```python
from build123d import *

# Parameters (mm, degrees)
SKETCH1_R           = 1.25
SKETCH1_R_2         = 1.75
BOSS_EXTRUDE2_DEPTH = 5


with BuildPart() as part:
    # Sketch1 → Boss-Extrude2 (new body)
    with BuildSketch(Plane.XY):
        with BuildLine():
            Line((386.419721239, 336.571497364), (385.293365012, 338.860526411))
            Line((385.293365012, 338.860526411), (383.908113185, 336.571143013))
            Line((383.908113185, 336.571143013), (382.503747201, 338.700952515))
            Line((382.503747201, 338.700952515), (381.416354322, 336.256003497))
            Line((381.416354322, 336.256003497), (379.756126272, 338.193005085))
            Line((379.756126272, 338.193005085), (378.983741177, 335.631048754))
            Line((378.983741177, 335.631048754), (377.093833849, 337.344694757))
            Line((377.093833849, 337.344694757), (376.648637512, 334.706134696))
            Line((376.648637512, 334.706134696), (374.558855873, 336.169399891))
            Line((374.558855873, 336.169399891), (374.447869306, 333.495847767))
            Line((374.447869306, 333.495847767), (372.191170461, 334.685655589))
            Line((372.191170461, 334.685655589), (372.41614399, 332.019274917))
            Line((372.41614399, 332.019274917), (370.028117427, 332.916861386))
            Line((370.028117427, 332.916861386), (370.585503084, 330.299702582))
            Line((370.585503084, 330.299702582), (368.10380941, 330.890912222))
            Line((368.10380941, 330.890912222), (368.98481689, 328.364249444))
            Line((368.98481689, 328.364249444), (366.448593896, 328.639758526))
            Line((366.448593896, 328.639758526), (367.639329184, 326.243438755))
            Line((367.639329184, 326.243438755), (365.088574622, 326.198902337))
            Line((365.088574622, 326.198902337), (366.570259113, 323.970716967))
            Line((366.570259113, 323.970716967), (364.045199905, 323.606837414))
            Line((364.045199905, 323.606837414), (365.794466549, 321.58192626))
            Line((365.794466549, 321.58192626), (363.334924388, 320.904442171))
            Line((363.334924388, 320.904442171), (365.324186205, 319.114739291))
            Line((365.324186205, 319.114739291), (362.96894954, 318.134334994))
            Line((362.96894954, 318.134334994), (365.166834682, 316.608065071))
            Line((365.166834682, 316.608065071), (362.953047003, 315.340202129))
            Line((362.953047003, 315.340202129), (365.324893508, 314.101435352))
            Line((365.324893508, 314.101435352), (363.287467569, 312.566108719))
            Line((363.287467569, 312.566108719), (365.795870002, 311.63438118))
            Line((365.795870002, 311.63438118), (363.966937226, 309.855803875))
            Line((363.966937226, 309.855803875), (366.572336582, 309.245809474))
            Line((366.572336582, 309.245809474), (364.980740332, 307.252030724))
            Line((364.980740332, 307.252030724), (367.642047906, 306.973389437))
            Line((367.642047906, 306.973389437), (366.312888606, 304.795852323))
            Line((366.312888606, 304.795852323), (368.988133989, 304.85295849))
            Line((368.988133989, 304.85295849), (367.942373274, 302.526004073))
            Line((367.942373274, 302.526004073), (370.589366248, 302.917957095))
            Line((370.589366248, 302.917957095), (369.84349639, 300.478282837))
            Line((369.84349639, 300.478282837), (372.420492294, 301.198901382))
            Line((372.420492294, 301.198901382), (371.986276106, 298.684982403))
            Line((371.986276106, 298.684982403), (374.452634175, 299.722901884))
            Line((374.452634175, 299.722901884), (374.336919507, 297.174384188))
            Line((374.336919507, 297.174384188), (376.653743801, 298.513235996))
            Line((376.653743801, 298.513235996), (376.85835554, 295.97031123))
            Line((376.85835554, 295.97031123), (378.989108357, 297.588980872))
            Line((378.989108357, 297.588980872), (379.510819655, 295.091752478))
            Line((379.510819655, 295.091752478), (379.666733337, 256.610886765))
            ThreePointArc((379.666733337, 256.610886765), (385.166733337, 251.110886765), (390.666733337, 256.610886765))
            Line((390.666733337, 256.610886765), (390.66667378, 256.636482058))
            Line((390.66667378, 256.636482058), (390.577340402, 295.028768444))
            Line((390.577340402, 295.028768444), (391.349725497, 297.590724775))
            Line((391.349725497, 297.590724775), (393.239632825, 295.877078772))
            Line((393.239632825, 295.877078772), (393.684829162, 298.515638833))
            Line((393.684829162, 298.515638833), (395.774610801, 297.052373638))
            Line((395.774610801, 297.052373638), (395.885597368, 299.725925762))
            Line((395.885597368, 299.725925762), (398.142296213, 298.53611794))
            Line((398.142296213, 298.53611794), (397.917322684, 301.202498612))
            Line((397.917322684, 301.202498612), (400.305349247, 300.304912143))
            Line((400.305349247, 300.304912143), (399.74796359, 302.922070947))
            Line((399.74796359, 302.922070947), (402.229657264, 302.330861307))
            Line((402.229657264, 302.330861307), (401.348649784, 304.857524085))
            Line((401.348649784, 304.857524085), (403.884872779, 304.582015003))
            Line((403.884872779, 304.582015003), (402.69413749, 306.978334774))
            Line((402.69413749, 306.978334774), (405.244892052, 307.022871192))
            Line((405.244892052, 307.022871192), (403.763207561, 309.251056562))
            Line((403.763207561, 309.251056562), (406.288266769, 309.614936115))
            Line((406.288266769, 309.614936115), (404.539000125, 311.639847269))
            Line((404.539000125, 311.639847269), (406.998542286, 312.317331358))
            Line((406.998542286, 312.317331358), (405.009280469, 314.107034238))
            Line((405.009280469, 314.107034238), (407.364517134, 315.087438535))
            Line((407.364517134, 315.087438535), (405.166631992, 316.613708458))
            Line((405.166631992, 316.613708458), (407.380419671, 317.8815714))
            Line((407.380419671, 317.8815714), (405.008573166, 319.120338177))
            Line((405.008573166, 319.120338177), (407.045999105, 320.65566481))
            Line((407.045999105, 320.65566481), (404.537596672, 321.587392349))
            Line((404.537596672, 321.587392349), (406.366529448, 323.365969654))
            Line((406.366529448, 323.365969654), (403.761130092, 323.975964055))
            Line((403.761130092, 323.975964055), (405.352726342, 325.969742805))
            Line((405.352726342, 325.969742805), (402.691418768, 326.248384092))
            Line((402.691418768, 326.248384092), (404.020578068, 328.425921206))
            Line((404.020578068, 328.425921206), (401.345332685, 328.368815039))
            Line((401.345332685, 328.368815039), (402.3910934, 330.695769456))
            Line((402.3910934, 330.695769456), (399.744100426, 330.303816434))
            Line((399.744100426, 330.303816434), (400.489970284, 332.743490692))
            Line((400.489970284, 332.743490692), (397.91297438, 332.022872147))
            Line((397.91297438, 332.022872147), (398.347190568, 334.536791126))
            Line((398.347190568, 334.536791126), (395.880832499, 333.498871645))
            Line((395.880832499, 333.498871645), (395.996547167, 336.047389341))
            Line((395.996547167, 336.047389341), (393.679722873, 334.708537533))
            Line((393.679722873, 334.708537533), (393.475111134, 337.251462299))
            Line((393.475111134, 337.251462299), (391.344358317, 335.632792657))
            Line((391.344358317, 335.632792657), (390.822647019, 338.130021051))
            Line((390.822647019, 338.130021051), (388.911568925, 336.257060962))
            Line((388.911568925, 336.257060962), (388.080985766, 338.6692102))
            Line((388.080985766, 338.6692102), (386.419721239, 336.571497364))
        make_face()
        with Locations((385.166733337, 256.610886765)):
            Circle(SKETCH1_R, mode=Mode.SUBTRACT)
        with Locations((385.166733337, 316.610886765)):
            Circle(SKETCH1_R_2, mode=Mode.SUBTRACT)
    extrude(amount=BOSS_EXTRUDE2_DEPTH)


solid = part.part
```
For this review, take the finished solid that the model builds, in its own axes (mm). Round coordinates to 2 decimals unless told otherwise and drop trailing zeros. Write each loop counter-clockwise with the first axis right and the second up, starting at its lowest first coordinate (ties: lowest second). Pieces come first, ordered by that corner, then holes.
1) Mouldability with a two-part tool opening along Y and no side actions: class faces 1 (the face through (401.795, 303.577, 2.465)), 2 (the face through (364.075, 315.983, 2.465)) as +Y half, -Y half, draft (parallel to the pull), parting line (faces both ways), or undercut.
Answer below:
face 1: undercut
face 2: undercut
2) Take a section at B-B on y = 263. Give the boundary of the cut face in (x, z).
Answer below:
outline: (379.64, 0) - (390.65, 0) - (390.65, 5) - (379.64, 5) - close
3) Take a section at A-A on z = 4.15. State how many separate pieces and enclosed holes the cut face has, then the cut area to 3 significant figures.
Answer below:
separate pieces: 1
enclosed holes: 2
area: 1,860 mm2
4) Take a section at C-C on y = 274. Give the boundary of the cut face in (x, z).
Answer below:
outline: (379.6, 0) - (390.63, 0) - (390.63, 5) - (379.6, 5) - close
5) For line 1 along Y through (x, z) = (367, 4.35); line 2 along X through (y, z) = (296.5, 1.15); line 3 along Y through (x, z) = (405.5, 4.2), list the stretches that pass through material, from the lowest coordinate up.
Answer below:
line 1: y = 304.81 to 305.92, 307.04 to 326.23, 327.53 to 328.58
line 2: x = 376.82 to 377.56, 379.22 to 391.02, 392.55 to 393.34
line 3: y = 309.5 to 310.53, 311.9 to 313.67, 314.31 to 316.38, 316.8 to 318.86, 319.49 to 321.23, 322.52 to 323.57
6) Insertion check: pin 1 Ø1 at (x, z) = (402.5, 3.5) entering from -Y; pin 2 Ø3 at (y, z) = (295, 1.5) entering from -X. Each pin has a flat end and moves straight along its axis. Give the tip position at first contact, or say it passes through.
Answer below:
pin 1: stops at y = 302.33
pin 2: stops at x = 376.82
